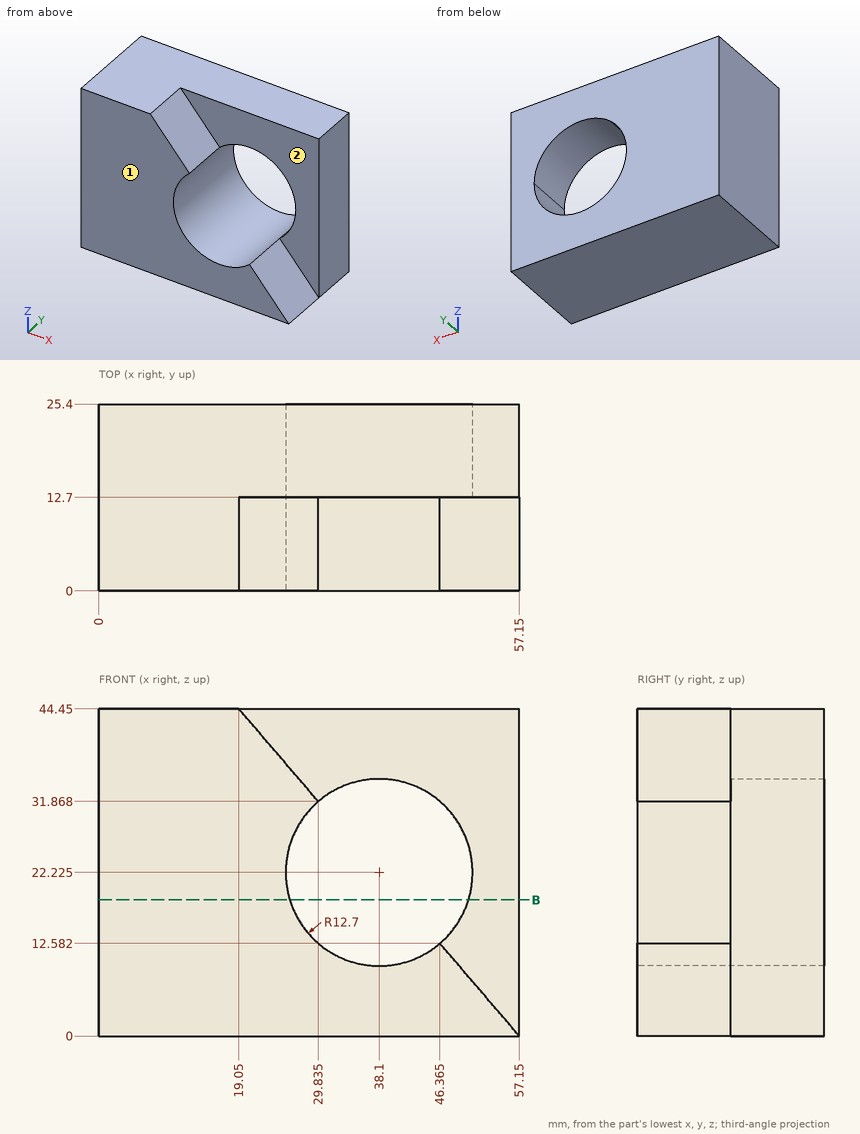
Design review of the part shown in the three views and the two pictorial views. Dimensions are in mm from the part's minimum x, y and z. A direction names the side the tool comes from. Give positions to 0.01 mm unless a question says otherwise; leave off trailing zeros. Loops run counter-clockwise (first coordinate to the right, second up) from the corner with the lowest first, then second, coordinate; pieces in that order, holes last. Notation, with made-up numbers: (71.5, 54) -> (107.5, 54) arc R14 ccw to (107.5, 60) -> close; hole circle Ø4 at (11, -36). An arc over 180 degrees is marked (long way). Put each result on its own line as item: value. Start each with the question number.
1. We need section B-B on z = 18.5. State the section outline as (x, y) points.
2. For the marked faces 1 and 2, list the 3-axis set-ups (+Z, -Z, +X, -X, +Y, -Y) from which the entire face can be reached by the end or side of a thin tool; tool diameter is ignored.
3. Clearance check with a flat-ended pin moving along its axis: P1, Ø2, axis at x = 38.5, y = 4, coming from the +Z side. State where the tip first meets the part, or that it passes through.
4. Wall thickness on probe 1 along Y at (x, z) = (40.5, 36); probe 2 along Z at (x, y) = (45, 13.5); probe 3 along X at (y, z) = (10, 22.5): over which ranges is each line inside the solid? List them lowest first.
Determined:
1. outline: (0, 0) -> (25.96, 0) -> (25.96, 25.4) -> (0, 25.4) -> close; (50.24, 12.7) -> (57.15, 12.7) -> (57.15, 25.4) -> (50.24, 25.4) -> close
2. face 1: +Z, -Z, +X, -X, -Y
2. face 2: +Z, +X, -Y
3. P1: z = 9.6
4. probe 1: 12.7 to 25.4
4. probe 2: 0 to 11.56, 32.89 to 44.45
4. probe 3: 0 to 25.4
